Design review of the part built by this model. Coordinates are the model's own, in mm. A direction names the side the tool comes from. Coordinates: 2 decimals unless noted, no trailing zeros. Loops run counter-clockwise (first coordinate to the right, second up) from the corner with the lowest first, then second, coordinate; pieces in that order, holes last. Notation, with made-up numbers: (72.25, 31.25) - (82.25, 31.25) arc R18 ccw to (82.25, 44.25) - close; hole circle Ø9 at (66, 21). An arc over 180 degrees is marked (long way). One line per question, with ' | ' between items.
from build123d import *

# Parameters (mm, degrees)
PAD_DEPTH    = 5
SKETCH001_R  = 1.5
PAD001_DEPTH = 8


with BuildPart() as part:
    # Sketch → Pad (new body)
    with BuildSketch(Plane.YZ):
        Polygon((-10.1, 0), (-8.1, 0), (-8.1, 2), (0, 2), (0, -10), (6, -10), (6, -14), (8, -14), (8, -10), (1.9, 4), (-10.1, 4), align=None)
    extrude(amount=PAD_DEPTH)

    # Sketch001 (on Face10 of Pad) → Pad001 (join)
    with BuildSketch(Plane.ZX.offset(8)):
        with Locations((-12, 2.5)):
            Circle(SKETCH001_R)
    extrude(amount=PAD001_DEPTH)


solid = part.part
Q1. Take a section at D-D (y = 0.5). Give the boundary of the cut face in (x, z).
Returned:
outline: (0, -10) - (5, -10) - (5, 4) - (0, 4) - close
Q2. Draft analysis for pull direction Y (two halves, no side actions). For faces 4 (the flat face through (3, 16, -12)), 5 (the cylindrical face through (1.6, 11.9, -13.2)), 6 (the flat face through (2, -10.1, 2)), 7 (the flat face through (2, -4, 2)), state which applies: +Y half, -Y half, draft (parallel to the pull), parting line (faces both ways), or undercut.
Returned:
face 4: +Y half | face 5: draft | face 6: -Y half | face 7: undercut
Q3. Take a section at C-C (y = -3.5). Give the boundary of the cut face in (x, z).
Returned:
outline: (0, 2) - (5, 2) - (5, 4) - (0, 4) - close
Q4. For pin 1 (1.5 mm diameter, centred on x = 2, y = -0.5, fed in from -Z); pin 2 (1.5 mm diameter, centred on x = 3.5, y = -4.5, fed in from -Z); pin 3 (2 mm diameter, centred on x = 3.5, z = -13, fed in from -Y), all flat-tipped, find the tip position at first contact; note any pin that passes through.
Returned:
pin 1: stops at z = -10 | pin 2: stops at z = 2 | pin 3: stops at y = 6
Q5. Take a section at A-A (x = 2.5). Give the boundary of the cut face in (y, z), plus the area to 4 significant figures.
Returned:
outline: (-10.1, 0) - (-8.1, 0) - (-8.1, 2) - (0, 2) - (0, -10) - (6, -10) - (6, -14) - (8, -14) - (8, -13.5) - (16, -13.5) - (16, -10.5) - (8, -10.5) - (8, -10) - (1.9, 4) - (-10.1, 4) - close | area: 125.5 mm²
Q6. To check wall thickness, follow line 1 along Y through (x, z) = (0.75, -11.5); line 2 along Z through (x, y) = (0.75, -4.5); line 3 along Z through (x, y) = (3.4, -8.25). State the ranges of each line that lie inside material, in increasing order.
Returned:
line 1: y = 6 to 8 | line 2: z = 2 to 4 | line 3: z = 0 to 4
Q7. Take a section at B-B (z = -12). Give the boundary of the cut face in (x, y).
Returned:
outline: (0, 6) - (5, 6) - (5, 8) - (4, 8) - (4, 16) - (1, 16) - (1, 8) - (0, 8) - close
Q8. Tool access review of faces 1 (the flat face through (0.8, 8, -12)), 2 (the flat face through (2, 0, -4)), 3 (the flat face through (2, 6, -12)): name each direction out of +Z, -Z, +X, -X, +Y, -Y from which nothing blocks a thin tool from reaching the whole face with its end or side.
Returned:
face 1: +Y | face 2: -Z, +X, -X | face 3: -Z, +X, -X, -Y
